from build123d import *

# Parameters (mm, degrees)
SKETCH1_R               = 13.75
BOSS_EXTRUDE1_DEPTH     = 2
SKETCH2_R               = 8.5
BOSS_EXTRUDE2_DEPTH     = 6
BOSS_EXTRUDE3_START     = 4
SKETCH3_R               = 13.75
BOSS_EXTRUDE3_DEPTH     = 2
SKETCH5_R               = 7
CUT_EXTRUDE2_DEPTH      = 21.350061425
BOSS_EXTRUDE4_START     = 6
SKETCH6_R               = 8.875
SKETCH6_R_2             = 7
BOSS_EXTRUDE4_DEPTH     = 5
CUT_EXTRUDE7_DEPTH      = 11
CUT_EXTRUDE7_DEPTH_BACK = 11
SKETCH17_R              = 0.25
CUT_EXTRUDE13_START     = 6
SKETCH16_R              = 0.25
CUT_EXTRUDE13_DEPTH     = 1


with BuildPart() as part:
    # Sketch1 → Boss-Extrude1 (new body)
    with BuildSketch(Plane.XY):
        Circle(SKETCH1_R)
    extrude(amount=BOSS_EXTRUDE1_DEPTH)

    # Sketch2 → Boss-Extrude2 (add)
    with BuildSketch(Plane.XY):
        Circle(SKETCH2_R)
    extrude(amount=BOSS_EXTRUDE2_DEPTH)

    # Sketch3 → Boss-Extrude3 (add)
    with BuildSketch(Plane.XY.offset(BOSS_EXTRUDE3_START)):
        Circle(SKETCH3_R)
    extrude(amount=BOSS_EXTRUDE3_DEPTH)

    # Sketch5 → Cut-Extrude2 (cut, through all)
    with BuildSketch(Plane.XY):
        Circle(SKETCH5_R)
    extrude(amount=CUT_EXTRUDE2_DEPTH, mode=Mode.SUBTRACT)

    # Sketch6 → Boss-Extrude4 (add)
    with BuildSketch(Plane.XY.offset(BOSS_EXTRUDE4_START)):
        Circle(SKETCH6_R)
        Circle(SKETCH6_R_2, mode=Mode.SUBTRACT)
    extrude(amount=BOSS_EXTRUDE4_DEPTH)

    # Sketch17 → Cut-Extrude7 (cut, two sides: drawn at the far end of the back side and taken through both)
    with BuildSketch(Plane(origin=(0, 0, 0), x_dir=(0, 0, -1), z_dir=(1, 0, 0)).offset(-CUT_EXTRUDE7_DEPTH_BACK)):
        with Locations(Location((-6.029707429, 0, 0), (0, 0, 180))):
            Circle(SKETCH17_R)
        with Locations(Location((-7.048386429, 0, 0), (0, 0, 180))):
            Circle(SKETCH17_R)
    extrude(amount=CUT_EXTRUDE7_DEPTH + CUT_EXTRUDE7_DEPTH_BACK, mode=Mode.SUBTRACT)

    # Sketch16 → Cut-Extrude13 (cut)
    with BuildSketch(Plane.XY.offset(CUT_EXTRUDE13_START)):
        with Locations((-7, 0)):
            Circle(SKETCH16_R)
        with Locations((7, 0)):
            Circle(SKETCH16_R)
    extrude(amount=CUT_EXTRUDE13_DEPTH, mode=Mode.SUBTRACT)


solid = part.part
Input: part model. Units: mm. Frame: model coordinates. A direction names the side the tool comes from. Round coordinates to 2 decimals unless told otherwise and drop trailing zeros. Write each loop counter-clockwise with the first axis right and the second up, starting at its lowest first coordinate (ties: lowest second). Pieces come first, ordered by that corner, then holes.
1) Reachability of faces 4 (the flat face through (0, -9, 4)), 5 (the flat face through (6, -6, 0)), 6 (the flat face through (3, -9, 6)) from +Z, -Z, +X, -X, +Y, -Y: full face, straight path, thin tool, end or side. Return the list, or none.
2) Cut plane C-C (z = 9.75). Return the cut outline in (x, y) (3 decimals).
3) Draft query along Y for faces 1 (the cylindrical face through (6.466, -2.681, 5.423)), 2 (the flat face through (0, -9, 2)), 3 (the cylindrical face through (-2.981, -13.423, 4.986)). Return one class per face: pulls with the +Y half, pulls with the -Y half, needs draft (parallel to the pull), parting line crosses it, or undercut.
4) Ray query, L1, parallel to Z at x = 9.95, y = 0; L2, parallel to Z at x = 9.5, y = 1.25; L3, parallel to X at y = -0.25, z = 3. Return the intervals inside material, ascending.
5) Cut plane D-D (y = 12). Return the cut outline in (x, z).
6) Cut plane A-A (x = 0). Return the cut outline in (y, z) (3 decimals).
7) Cut plane B-B (y = -2.5). Return the cut outline in (x, z), then the cut area to 3 significant figures.
8) Contact query for flat-ended pins moving along their axis: P1, Ø6, axis at x = 5.5, z = 8.5, coming from the +Y side; P2, Ø1, axis at y = 2, z = 6, coming from the +X side; P3, Ø12.5, axis at x = 0, y = 0, coming from the -Z side; P4, Ø1, axis at y = -11, z = 6, coming from the +X side. Output: stop coordinate, or through.
Geometry says:
1. face 4: none
1. face 5: -Z, +X, -X, +Y, -Y
1. face 6: +Z
2. outline: circle Ø17.75 at (0, 0); hole circle Ø14 at (0, 0)
3. face 1: undercut
3. face 2: needs draft
3. face 3: parting line crosses it
4. L1: z = 0 to 2, 4 to 5.78
4. L2: z = 0 to 2, 4 to 6
4. L3: x = -8.5 to -7, 7 to 8.5
5. outline: (-6.71, 0) - (6.71, 0) - (6.71, 2) - (-6.71, 2) - close; (-6.71, 4) - (6.71, 4) - (6.71, 6) - (-6.71, 6) - close
6. outline: (-13.75, 0) - (-7, 0) - (-7, 11) - (-8.875, 11) - (-8.875, 6) - (-13.75, 6) - (-13.75, 4) - (-8.5, 4) - (-8.5, 2) - (-13.75, 2) - close; (7, 0) - (13.75, 0) - (13.75, 2) - (8.5, 2) - (8.5, 4) - (13.75, 4) - (13.75, 6) - (8.875, 6) - (8.875, 11) - (7, 11) - close
7. outline: (-13.52, 0) - (-6.54, 0) - (-6.54, 11) - (-8.52, 11) - (-8.52, 6) - (-13.52, 6) - (-13.52, 4) - (-8.12, 4) - (-8.12, 2) - (-13.52, 2) - close; (6.54, 0) - (13.52, 0) - (13.52, 2) - (8.12, 2) - (8.12, 4) - (13.52, 4) - (13.52, 6) - (8.52, 6) - (8.52, 11) - (6.54, 11) - close
7. area: 82.0 mm2
8. P1: stops at y = 13.2
8. P2: stops at x = 13.67
8. P3: passes through
8. P4: stops at x = 8.88
